Check sheet for the modelled part. Datum: model origin and axes. Units: mm. Face numbers are marked on the shaded views. A direction names the side the tool comes from. Coordinates: 2 decimals unless noted, no trailing zeros. Loops run counter-clockwise (first coordinate to the right, second up) from the corner with the lowest first, then second, coordinate; pieces in that order, holes last.
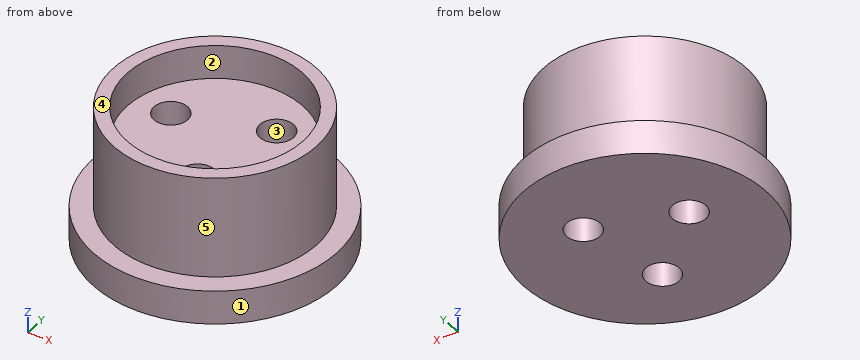
from build123d import *

# Parameters (mm, degrees)
SKETCH1_R           = 18
SKETCH1_R_2         = 15
BOSS_EXTRUDE1_DEPTH = 5
SKETCH1_3_R         = 15
SKETCH1_3_R_2       = 13
BOSS_EXTRUDE2_DEPTH = 20
SKETCH1_4_R         = 13
BOSS_EXTRUDE3_DEPTH = 15
SKETCH2_R           = 2.5
CUT_EXTRUDE1_DEPTH  = 30.546573405


with BuildPart() as part:
    # Sketch1 → Boss-Extrude1 (new body)
    with BuildSketch(Plane.XY):
        Circle(SKETCH1_R)
        Circle(SKETCH1_R_2, mode=Mode.SUBTRACT)
    extrude(amount=BOSS_EXTRUDE1_DEPTH)

    # Sketch1<3> → Boss-Extrude2 (add)
    with BuildSketch(Plane.XY):
        Circle(SKETCH1_3_R)
        Circle(SKETCH1_3_R_2, mode=Mode.SUBTRACT)
    extrude(amount=BOSS_EXTRUDE2_DEPTH)

    # Sketch1<4> → Boss-Extrude3 (add)
    with BuildSketch(Plane.XY):
        Circle(SKETCH1_4_R)
    extrude(amount=BOSS_EXTRUDE3_DEPTH)

    # Sketch2 → Cut-Extrude1 (cut, through all)
    with BuildSketch(Plane.XY.offset(15)):
        with Locations((-7.66, 1.666394077)):
            Circle(SKETCH2_R)
        with Locations((5.273139603, 5.800557555)):
            Circle(SKETCH2_R)
        with Locations((2.386860397, -7.466951631)):
            Circle(SKETCH2_R)
    extrude(amount=-CUT_EXTRUDE1_DEPTH, mode=Mode.SUBTRACT)


solid = part.part
(1) Set-up check for the marked faces 1 and 2: record each of +Z, -Z, +X, -X, +Y, -Y from which the full face is reachable in a straight line by a thin tool's end or side.
(2) Section check A-A, the plane y = 7.5. Enter the section's corners in (x, z), plus the area to 3 significant figures.
(3) Section check B-B, the plane x = -7.66. Enter the section's corners in (y, z), plus the area to 3 significant figures.
(4) Gauge pin test, flat ends, axial feed: P1, Ø3, axis at y = 11, z = 9.5, coming from the -X side; P2, Ø5, axis at x = -3, z = 4.5, coming from the -Y side; P3, Ø1, axis at y = 14, z = 2.5, coming from the -X side. Record the tip position at first contact, or that the pin passes through.
(5) Section check D-D, the plane x = -1.5. Enter the section's corners in (y, z).
(6) Scan lines: line 1 along Y through (x, z) = (3, 7.5); line 2 along Y through (x, z) = (-0.5, 8.75); line 3 along Z through (x, y) = (-8, 7.5). Record each from-to range of solid material in increasing order.
(7) Draft check along X on the marked faces 3, 4 and 5. Enter one of: pulls with the +X half, pulls with the -X half, needs draft (parallel to the pull), parting line crosses it, or undercut.
(8) Section check C-C, the plane z = 15.5. Enter the section's corners in (x, y), plus the area to 3 significant figures.
Determined:
1. face 1: +Z, -Z
1. face 2: +Z
2. outline: (-16.36, 0) - (3.44, 0) - (3.44, 15) - (-10.62, 15) - (-10.62, 20) - (-12.99, 20) - (-12.99, 5) - (-16.36, 5) - close; (7.11, 0) - (16.36, 0) - (16.36, 5) - (12.99, 5) - (12.99, 20) - (10.62, 20) - (10.62, 15) - (7.11, 15) - close
2. area: 392 mm2
3. outline: (-16.29, 0) - (-0.83, 0) - (-0.83, 15) - (-10.5, 15) - (-10.5, 20) - (-12.9, 20) - (-12.9, 5) - (-16.29, 5) - close; (4.17, 0) - (16.29, 0) - (16.29, 5) - (12.9, 5) - (12.9, 20) - (10.5, 20) - (10.5, 15) - (4.17, 15) - close
3. area: 370 mm2
4. P1: stops at x = -11.61
4. P2: stops at y = -17.99
4. P3: stops at x = -11.91
5. outline: (-17.94, 0) - (17.94, 0) - (17.94, 5) - (14.92, 5) - (14.92, 20) - (12.91, 20) - (12.91, 15) - (-12.91, 15) - (-12.91, 20) - (-14.92, 20) - (-14.92, 5) - (-17.94, 5) - close
6. line 1: y = -14.7 to -9.89, -5.04 to 4.76, 6.84 to 14.7
6. line 2: y = -14.99 to 14.99
6. line 3: z = 0 to 15
7. face 3: undercut
7. face 4: needs draft
7. face 5: parting line crosses it
8. outline: circle Ø30 at (0, 0); hole circle Ø26 at (0, 0)
8. area: 176 mm2
